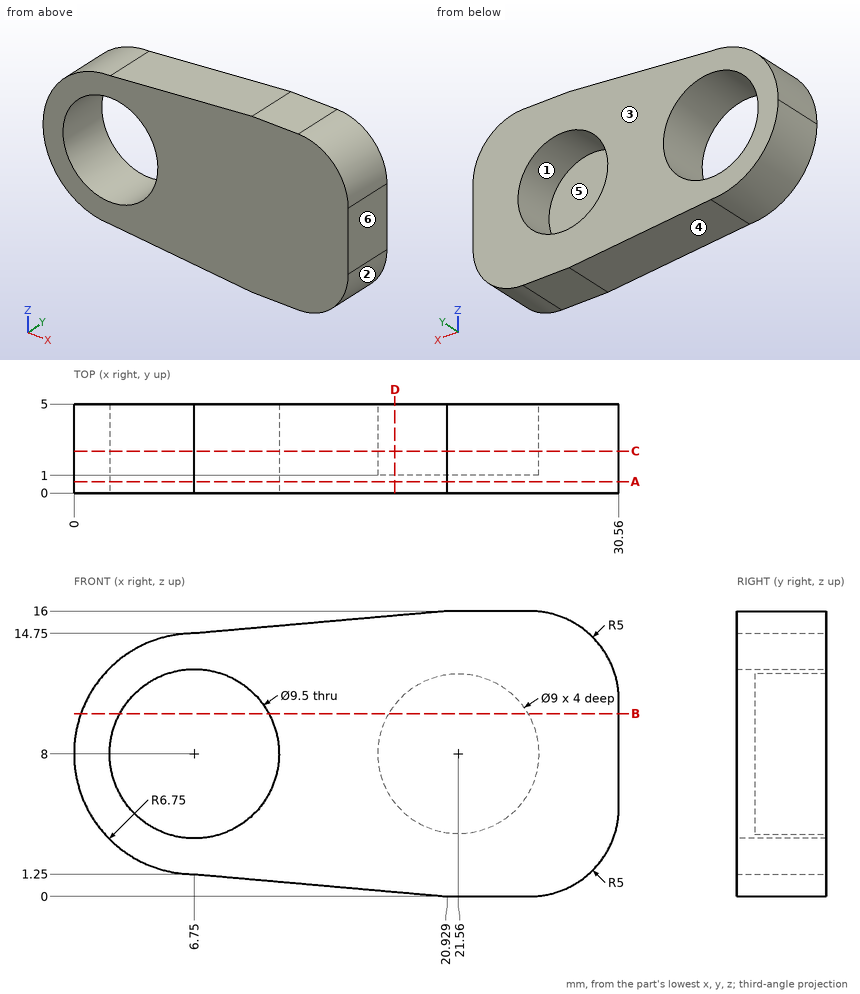
Print and shaded views of the part. All mm, measured from the part's lowest x, y and z. A direction names the side the tool comes from. Round coordinates to 2 decimals unless told otherwise and drop trailing zeros. Write each loop counter-clockwise with the first axis right and the second up, starting at its lowest first coordinate (ties: lowest second). Pieces come first, ordered by that corner, then holes. Notation, with made-up numbers: (32, 81) - (70, 81) arc R3 ccw to (70, 86) - close; hole circle Ø9 at (62, -18.5). An arc over 180 degrees is marked (long way). One line per item, written item: value.
(1) Two-plate mould, pull along X, no slides. Class the marked faces 1, 2, 3 and 4: pulls with the +X half, pulls with the -X half, needs draft (parallel to the pull), parting line crosses it, or undercut.
Values follow:
face 1: undercut
face 2: pulls with the +X half
face 3: needs draft
face 4: pulls with the -X half
(2) Cut at C-C, the plane y = 2.35. Give the cut face in (x, z).
Values follow:
outline: (0, 8) arc R6.75 ccw to (6.75, 1.25) - (20.93, 0) - (25.56, 0) arc R5 ccw to (30.56, 5) - (30.56, 11) arc R5 ccw to (25.56, 16) - (20.93, 16) - (6.75, 14.75) arc R6.75 ccw to start; hole circle Ø9.5 at (6.75, 8); hole circle Ø9 at (21.56, 8)
(3) Drop flat-ended pins along their axis: P1, Ø8, axis at x = 21.56, z = 8, coming from the +Y side; P2, Ø8.5, axis at x = 6.75, z = 8, coming from the -Y side (3 decimals); P3, Ø5, axis at x = 17, z = 5.5, coming from the -Y side. Give the stop position or say it passes through.
Values follow:
P1: stops at y = 1
P2: passes through
P3: stops at y = 0
(4) Cut at B-B, the plane z = 10.25. Give the cut face in (x, y).
Values follow:
outline: (0.39, 0) - (2.57, 0) - (2.57, 5) - (0.39, 5) - close; (10.93, 0) - (30.56, 0) - (30.56, 5) - (25.46, 5) - (25.46, 1) - (17.66, 1) - (17.66, 5) - (10.93, 5) - close
(5) 3-axis set-ups, long thin cutter, end or side, ignore diameter. For the marked faces 5 and 6: which of +Z, -Z, +X, -X, +Y, -Y reach the whole face in a straight line?
Values follow:
face 5: +Y
face 6: +Z, -Z, +X, +Y, -Y
(6) Wall check: probe 1 along X at (y, z) = (3.35, 8); probe 2 along X at (y, z) = (4.3, 11.75) (1 decimal); probe 3 along Z at (x, y) = (6.5, 3.35). Give the ranges that are in metal, low to high.
Values follow:
probe 1: x = 0 to 2, 11.5 to 17.06, 26.06 to 30.56
probe 2: x = 1.1 to 3.8, 9.7 to 19.1, 24 to 30.5
probe 3: z = 1.25 to 3.26, 12.74 to 14.75
(7) Cut at D-D, the plane x = 18. Give the cut face in (y, z), plus the area to 3 significant figures.
Values follow:
outline: (0, 0.26) - (5, 0.26) - (5, 5.25) - (1, 5.25) - (1, 10.75) - (5, 10.75) - (5, 15.74) - (0, 15.74) - close
area: 55.4 mm²
(8) Cut at A-A, the plane y = 0.65. Give the cut face in (x, z).
Values follow:
outline: (0, 8) arc R6.75 ccw to (6.75, 1.25) - (20.93, 0) - (25.56, 0) arc R5 ccw to (30.56, 5) - (30.56, 11) arc R5 ccw to (25.56, 16) - (20.93, 16) - (6.75, 14.75) arc R6.75 ccw to start; hole circle Ø9.5 at (6.75, 8)
